Here's how the part is built. I have some questions about the finished solid (model axes, mm). Face numbers are marked on the shaded views. A direction names the side the tool comes from. Coordinates: 2 decimals unless noted, no trailing zeros. Write each loop counter-clockwise with the first axis right and the second up, starting at its lowest first coordinate (ties: lowest second). Pieces come first, ordered by that corner, then holes. Notation, with made-up numbers: M 52.5,84.25 L 57.5,84.25 A23 ccw 57.5,95.25 Z; hole C -1,-3 d5. An arc over 180 degrees is marked long. Use a Markdown table: item, result.
```python
from build123d import *

# Parameters (mm, degrees)
ESQUISSE2_W              = 100
ESQUISSE2_H              = 50
BOSS_EXTRU_1_DEPTH       = 50
ENL_V_MAT_EXTRU_2_DEPTH  = 51
ESQUISSE7_W              = 40
ESQUISSE7_H              = 50
ENL_V_MAT_EXTRU_3_DEPTH  = 20
ESQUISSE8_W              = 30
ESQUISSE8_H              = 30
ENL_V_MAT_EXTRU_4_DEPTH  = 20
ENL_V_MAT_EXTRU_7_DEPTH  = 2.5
ENL_V_MAT_EXTRU_10_DEPTH = 5
ENL_V_MAT_EXTRU_11_DEPTH = 5
ENL_V_MAT_EXTRU_12_DEPTH = 10
ESQUISSE16_R             = 17.5
ESQUISSE16_R_2           = 15
ENL_V_MAT_EXTRU_13_DEPTH = 2.5
ESQUISSE17_R             = 12
ENL_V_MAT_EXTRU_14_DEPTH = 2.5


with BuildPart() as part:
    # Esquisse2 → Boss.-Extru.1 (new body)
    with BuildSketch(Plane.XY):
        with Locations((19.891640867, -6.114551084)):
            Rectangle(ESQUISSE2_W, ESQUISSE2_H)
    extrude(amount=BOSS_EXTRU_1_DEPTH)

    # Esquisse5 → Enlèv. mat.-Extru.2 (cut, through all)
    with BuildSketch(Plane(origin=(0, -31.114551084, 0), x_dir=(-1, 0, 0), z_dir=(0, -1, 0))):
        Polygon((30.108359133, 0), (20.108359133, -10), (20.108359133, -50), (30.108359133, -50), align=None)
        Polygon((-69.891640867, 0), (-59.891640867, -10), (-59.891640867, -50), (-69.891640867, -50), align=None)
    extrude(amount=-ENL_V_MAT_EXTRU_2_DEPTH, mode=Mode.SUBTRACT)

    # Esquisse7 → Enlèv. mat.-Extru.3 (cut)
    with BuildSketch(Plane.XY.offset(50)):
        with Locations((39.891640867, -6.114551084)):
            Rectangle(ESQUISSE7_W, ESQUISSE7_H)
    extrude(amount=-ENL_V_MAT_EXTRU_3_DEPTH, mode=Mode.SUBTRACT)

    # Esquisse8 → Enlèv. mat.-Extru.4 (cut)
    with BuildSketch(Plane.XY.offset(50)):
        with Locations((4.891640867, -6.114551084)):
            Rectangle(ESQUISSE8_W, ESQUISSE8_H)
    extrude(amount=-ENL_V_MAT_EXTRU_4_DEPTH, mode=Mode.SUBTRACT)

    # Esquisse9 → Enlèv. mat.-Extru.7 (cut)
    with BuildSketch(Plane.XY.offset(30)):
        with BuildLine():
            Line((25.877762678, 8.885448916), (19.891640867, 8.885448916))
            Line((19.891640867, 8.885448916), (-10.108359133, 8.885448916))
            Line((-10.108359133, 8.885448916), (-10.108359133, -20.265562259))
            Line((-10.108359133, -20.265562259), (-10.108359133, -21.114551084))
            Line((-10.108359133, -21.114551084), (19.891640867, -21.114551084))
            Line((19.891640867, -21.114551084), (26.628394236, -21.540787019))
            ThreePointArc((26.628394236, -21.540787019), (17.396963997, -6.546154144), (25.877762678, 8.885448916))
        make_face()
    extrude(amount=-ENL_V_MAT_EXTRU_7_DEPTH, mode=Mode.SUBTRACT)

    # Esquisse11 → Enlèv. mat.-Extru.10 (cut)
    with BuildSketch(Plane.XY.offset(30)):
        with BuildLine():
            Line((26.628394236, -21.540787019), (19.891640867, -21.114551084))
            Line((19.891640867, -21.114551084), (19.891640867, -31.114551084))
            Line((19.891640867, -31.114551084), (59.891640867, -31.114551084))
            Line((59.891640867, -31.114551084), (59.891640867, 18.885448916))
            Line((59.891640867, 18.885448916), (19.891640867, 18.885448916))
            Line((19.891640867, 18.885448916), (19.891640867, 8.885448916))
            Line((19.891640867, 8.885448916), (25.877762678, 8.885448916))
            ThreePointArc((25.877762678, 8.885448916), (43.508691746, 9.116878073), (52.391640867, -6.114551084))
            ThreePointArc((52.391640867, -6.114551084), (43.881723847, -21.12882456), (26.628394236, -21.540787019))
        make_face()
    extrude(amount=-ENL_V_MAT_EXTRU_10_DEPTH, mode=Mode.SUBTRACT)

    # Esquisse13 → Enlèv. mat.-Extru.11 (cut)
    with BuildSketch(Plane.XY.offset(30)):
        with BuildLine():
            ThreePointArc((26.628394236, -21.540787019), (17.396963997, -6.546154144), (25.877762678, 8.885448916))
            Line((25.877762678, 8.885448916), (-10.108359133, 8.885448916))
            Line((-10.108359133, 8.885448916), (-10.108359133, -21.114551084))
            Line((-10.108359133, -21.114551084), (26.628394236, -21.540787019))
        make_face()
    extrude(amount=-ENL_V_MAT_EXTRU_11_DEPTH, mode=Mode.SUBTRACT)

    # Esquisse15 → Enlèv. mat.-Extru.12 (cut)
    with BuildSketch(Plane(origin=(0, -31.114551084, 0), x_dir=(-1, 0, 0), z_dir=(0, -1, 0))):
        Polygon((10.108359133, -50), (-19.891640867, -25), (-19.891640867, -50), align=None)
    extrude(amount=-ENL_V_MAT_EXTRU_12_DEPTH, mode=Mode.SUBTRACT)

    # Esquisse16 → Enlèv. mat.-Extru.13 (cut)
    with BuildSketch(Plane.XY.offset(30)):
        with Locations((34.891640867, -6.114551084)):
            Circle(ESQUISSE16_R)
        with Locations((34.891640867, -6.114551084)):
            Circle(ESQUISSE16_R_2, mode=Mode.SUBTRACT)
    extrude(amount=-ENL_V_MAT_EXTRU_13_DEPTH, mode=Mode.SUBTRACT)

    # Esquisse17 → Enlèv. mat.-Extru.14 (cut)
    with BuildSketch(Plane.XY.offset(30)):
        with Locations((34.891640867, -6.114551084)):
            Circle(ESQUISSE17_R)
    extrude(amount=-ENL_V_MAT_EXTRU_14_DEPTH, mode=Mode.SUBTRACT)


solid = part.part
```
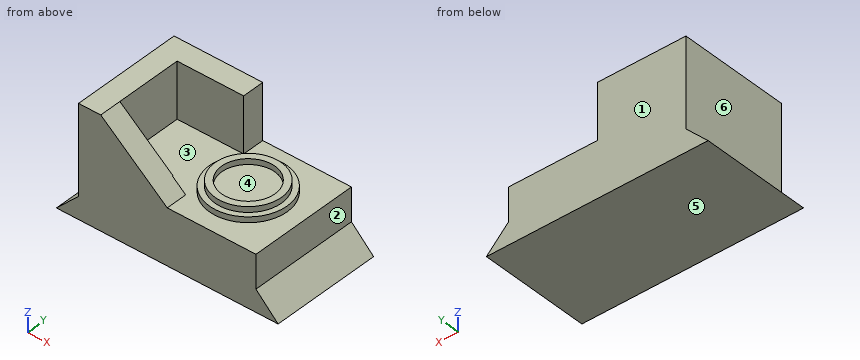
1. Will these pins go through, and if not, where does the flat tip stop? pin 1 Ø8 at (y, z) = (13, 42) entering from +X; pin 2 Ø5 at (y, z) = (-18.5, 30.5) entering from +X; pin 3 Ø16.5 at (y, z) = (-4, 16.5) entering from +X; pin 4 Ø20 at (x, z) = (11, 35) entering from -Y.
Answers follow:
| item | result |
|---|---|
| pin 1 | stops at x = 19.89 |
| pin 2 | stops at x = 46.13 |
| pin 3 | stops at x = 61.64 |
| pin 4 | stops at y = -31.11 |
2. Which directions (+Z, -Z, +X, -X, +Y, -Y) give clear straight access to the entire face, cutting with the end or side of a thin tool? Please do the marked faces 4, 5 and 6.
Answers follow:
| item | result |
|---|---|
| face 4 | +Z |
| face 5 | -Z, +X, -X, +Y, -Y |
| face 6 | +Z, -X, +Y, -Y |
3. We'd pull the mould along X, two halves only. Please class the marked faces 1, 2 and 3: +X half, -X half, draft (parallel to the pull), parting line (faces both ways), or undercut.
Answers follow:
| item | result |
|---|---|
| face 1 | draft |
| face 2 | +X half |
| face 3 | undercut |
4. I need wall thicknesses on probe 1 along Y at (x, z) = (11, 31.5); probe 2 along X at (y, z) = (-2.5, 16.5); probe 3 along X at (y, z) = (-1, 40.5). Which ranges of each line are inside material? Lowest first, please.
Answers follow:
| item | result |
|---|---|
| probe 1 | y = -31.11 to -21.11, 8.89 to 18.89 |
| probe 2 | x = -20.11 to 59.89 |
| probe 3 | x = -20.11 to -10.11 |
5. Suppose I cut it at B-B on z = 31.5. Write out the boundary of the cut face in (x, y), and give its area (3 significant figures).
Answers follow:
| item | result |
|---|---|
| outline | M -20.11,-31.11 L 12.09,-31.11 L 12.09,-21.11 L -10.11,-21.11 L -10.11,8.89 L 19.89,8.89 L 19.89,18.89 L -20.11,18.89 Z |
| area | 1,020 mm2 |
6. Suppose I cut it at A-A on x = 11.5. Write out the boundary of the cut face in (y, z).
Answers follow:
| item | result |
|---|---|
| outline | M -31.11,0 L 18.89,0 L 18.89,50 L 8.89,50 L 8.89,25 L -21.37,25 L -21.37,30 L -21.11,30 L -21.11,31.99 L -31.11,31.99 Z |
7. Suppose I cut it at C-C on y = 2.5. Write out the boundary of the cut face in (x, z), and give its area (3 significant figures).
Answers follow:
| item | result |
|---|---|
| outline | M -30.11,0 L 69.89,0 L 59.89,10 L 59.89,25 L 50.12,25 L 50.12,27.5 L 47.17,27.5 L 47.17,30 L 43.25,30 L 43.25,27.5 L 26.54,27.5 L 26.54,30 L 22.61,30 L 22.61,27.5 L 19.66,27.5 L 19.66,25 L -10.11,25 L -10.11,50 L -20.11,50 L -20.11,10 Z |
| area | 2,450 mm2 |
